Part print with two shaded views. Sizes in mm from the minimum x, y, z corner. A direction names the side the tool comes from. Give positions to 0.01 mm unless a question says otherwise; leave off trailing zeros. Write each loop counter-clockwise with the first axis right and the second up, starting at its lowest first coordinate (ties: lowest second). Pieces come first, ordered by that corner, then holes.
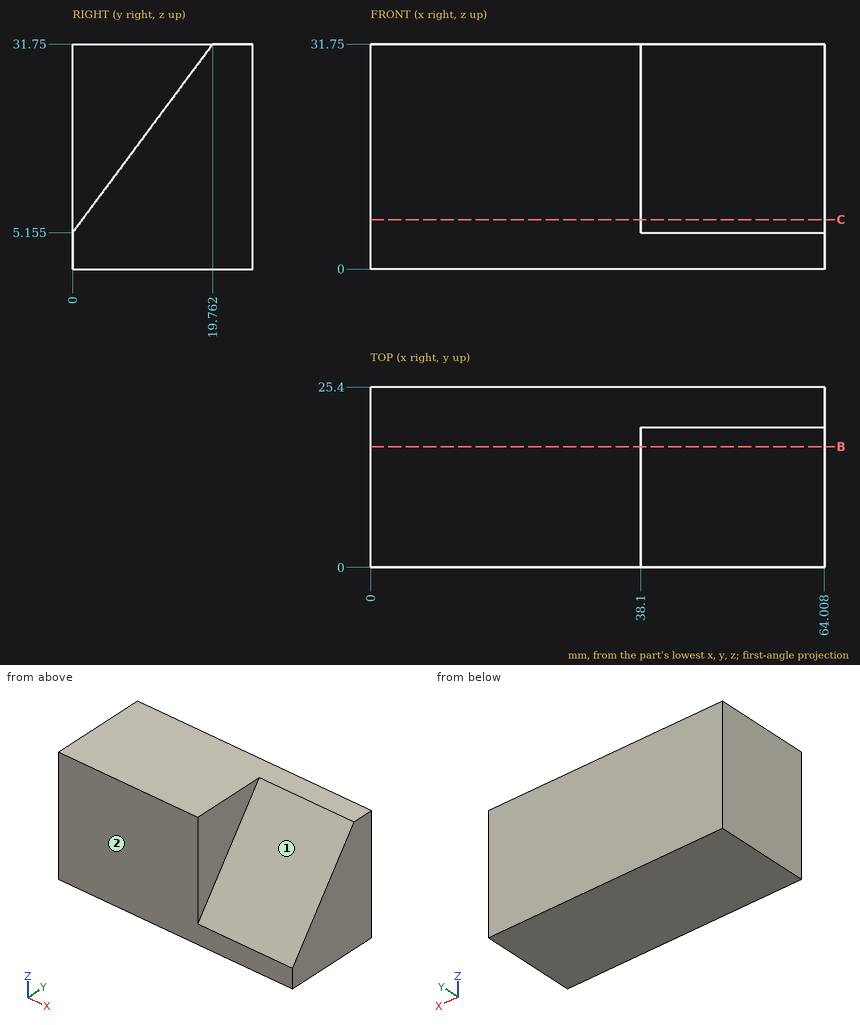
1) Flat gauge pin, fed straight in: P1, Ø6, axis at y = 10, z = 24, coming from the +X side. Where does the tip first touch, or does it go through?
Check result:
P1: stops at x = 38.1
2) 3-axis set-ups, long thin cutter, end or side, ignore diameter. For the marked faces 1 and 2: which of +Z, -Z, +X, -X, +Y, -Y reach the whole face in a straight line?
Check result:
face 1: +Z, +X, -Y
face 2: +Z, -Z, +X, -X, -Y
3) Saw through at C-C (z = 7). Write the cut outline in (x, y).
Check result:
outline: (0, 0) - (38.1, 0) - (38.1, 1.37) - (64.01, 1.37) - (64.01, 25.4) - (0, 25.4) - close
4) Saw through at B-B (y = 17). Write the cut outline in (x, z).
Check result:
outline: (0, 0) - (64.01, 0) - (64.01, 28.03) - (38.1, 28.03) - (38.1, 31.75) - (0, 31.75) - close
5) Drill centre lines: L1, parallel to X at y = 1.75, z = 20.5; L2, parallel to Y at x = 47.5, z = 9.5; L3, parallel to Z at x = 46, y = 7.25. Where is each one in solid material? Low to high.
Check result:
L1: x = 0 to 38.1
L2: y = 3.23 to 25.4
L3: z = 0 to 14.91
